Geometry check sheet. Reference: the model listing, model coordinates, mm. Face numbers are marked on the shaded views. A direction names the side the tool comes from. Give positions to 0.01 mm unless a question says otherwise; leave off trailing zeros. Order: outer loops, then holes, each group sorted by start corner. A loop starts at its lowest first (then second) coordinate and runs counter-clockwise, first axis right, second up. Notation, with made-up numbers: M -33.75,-29.75 L -19.75,-29.75 A12 ccw -19.75,-14.75 Z; hole C -25.75,-2.75 d2. An arc over 180 degrees is marked long. Answer as CSV lines item,"result".
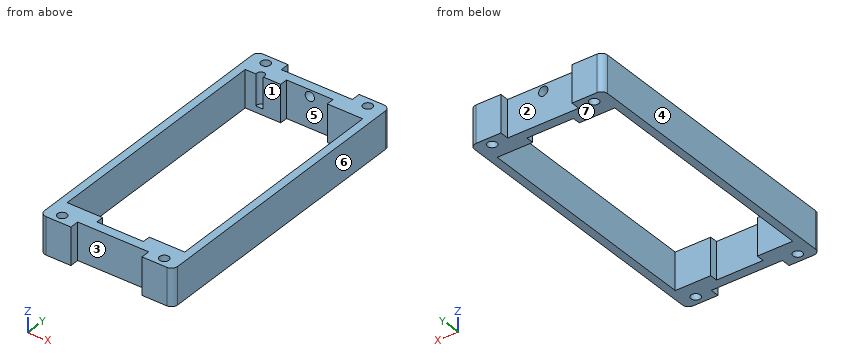
Autodesk Inventor part; units mm, degrees
ref_plane "YZ Plane" through (0, 0, 0) normal (1, 0, 0) x (0, 1, 0)
ref_plane "XZ Plane" through (0, 0, 0) normal (0, 1, 0) x (-1, 0, 0)
ref_plane "XY Plane" through (0, 0, 0) normal (0, 0, 1) x (1, 0, 0)
sketch "Эскиз1" plane through (0, 0, 0) normal (0, 0, 1) x (1, 0, 0)
  line L0 (-18.25, -37.6) -> (18.25, -37.6)
  line L1 (18.25, -37.6) -> (18.25, 37.6)
  line L2 (18.25, 37.6) -> (-18.25, 37.6)
  line L3 (-18.25, 37.6) -> (-18.25, -37.6)
  line L4 (-18.25, 0) -> (18.25, 0) construction
  line L5 (0, 37.6) -> (0, -37.6) construction
  line L6 (-18.45, -37.8) -> (18.45, -37.8)
  line L7 (18.45, -37.8) -> (18.45, 37.8)
  line L8 (18.45, 37.8) -> (-18.45, 37.8)
  line L9 (-18.45, 37.8) -> (-18.45, -37.8)
  line L10 (-7.5, -37.8) -> (7.5, -37.8)
  line L11 (7.5, -37.8) -> (7.5, -40.8)
  line L12 (7.5, -40.8) -> (-7.5, -40.8)
  line L13 (-7.5, -40.8) -> (-7.5, -37.8)
  line L14 (-18.45, -37.8) -> (-18.45, -43.8)
  line L15 (-18.45, -43.8) -> (18.45, -43.8)
  line L16 (18.45, -43.8) -> (18.45, -37.8)
  line L17 (-18.45, 43.8) -> (18.45, 43.8)
  line L18 (-18.45, 37.8) -> (-18.45, 43.8)
  line L19 (18.45, 43.8) -> (18.45, 37.8)
  line L20 (-18.45, -43.8) -> (-21.45, -43.8)
  line L21 (-21.45, -43.8) -> (-21.45, 43.8)
  line L22 (-21.45, 43.8) -> (-18.45, 43.8)
  line L23 (-18.45, 43.8) -> (-18.45, -43.8)
  line L24 (21.45, 43.8) -> (18.45, 43.8)
  line L25 (18.45, 37.8) -> (18.45, 43.8)
  line L26 (18.45, 43.8) -> (18.45, -43.8)
  line L27 (21.45, -43.8) -> (21.45, 43.8)
  line L28 (-7.5, 40.8) -> (-7.5, 37.8)
  line L29 (7.5, 40.8) -> (-7.5, 40.8)
  line L30 (7.5, 37.8) -> (7.5, 40.8)
  line L31 (-21.45, -43.8) -> (-11.45, -43.8)
  line L32 (18.45, -43.8) -> (21.45, -43.8)
  line L33 (21.45, -43.8) -> (11.45, -43.8)
  line L34 (16.45, 46.7) -> (21.45, 46.7)
  line L35 (16.45, 46.7) -> (11.45, 46.7)
  line L36 (11.45, 46.7) -> (11.45, 43.8)
  line L37 (21.45, 46.7) -> (21.45, 43.8)
  line L38 (11.45, 43.8) -> (16.45, 43.8)
  line L39 (-11.45, 46.7) -> (-11.45, 43.8)
  line L40 (-16.45, 46.7) -> (-11.45, 46.7)
  line L41 (-16.45, 46.7) -> (-21.45, 46.7)
  line L42 (-21.45, 46.7) -> (-21.45, 43.8)
  line L43 (-16.45, -46.7) -> (-21.45, -46.7)
  line L44 (-21.45, -46.7) -> (-21.45, -43.8)
  line L45 (-16.45, -46.7) -> (-11.45, -46.7)
  line L46 (-11.45, -46.7) -> (-11.45, -43.8)
  line L47 (11.45, -46.7) -> (11.45, -43.8)
  line L48 (16.45, -46.7) -> (11.45, -46.7)
  line L49 (16.45, -46.7) -> (21.45, -46.7)
  line L50 (21.45, -46.7) -> (21.45, -43.8)
  circle A0 centre (16.45, -43.8) radius 1.5
  circle A1 centre (-16.45, -43.8) radius 1.5
  circle A2 centre (16.45, 43.8) radius 1.5
  circle A3 centre (-16.45, 43.8) radius 1.5
  line L51 (0, 0) -> (-14.3, 0) construction
  line L52 (-14.3, 0) -> (-14.3, 38.8) construction
  line L53 (-14.3, 38.8) -> (0, 38.8) construction
  line L54 (0, 38.8) -> (0, 0) construction
  circle A4 centre (-14.3, 38.8) radius 1.25
  line L55 (18.45, -37.8) -> (18.95, -37.8)
  line L56 (18.95, -37.8) -> (18.95, -38.3)
  line L57 (18.95, -38.3) -> (18.45, -38.3)
  line L58 (18.45, -38.3) -> (18.45, -37.8)
  line L59 (18.95, -38.3) -> (-18.95, -38.3)
  line L60 (-18.95, -38.3) -> (-18.95, 38.3)
  line L61 (-18.95, 38.3) -> (18.95, 38.3)
  line L62 (18.95, 38.3) -> (18.95, -38.3)
  point P0 (-1.9914, -32.8601)
  point P1 (0, -37.8)
  point P2 (-15.05, 37.8)
  point P3 (-13.55, 37.8)
  point P4 (7.5, -38.3)
  point P5 (-7.5, -38.3)
  point P6 (-7.5, 38.3)
  point P7 (7.5, 38.3)
  dimension "d0" = 36.5
  dimension "d1" = 75.2
  dimension "d2" = 36.9
  dimension "d3" = 75.6
  dimension "d4" = 15
  dimension "d5" = 3
  dimension "d6" = 6
  dimension "d7" = 3
  dimension "d8" = 5
  dimension "d10" = 3
  dimension "d11" = 3
  dimension "d12" = 3
  dimension "d13" = 3
  dimension "d19" = 14.3
  dimension "d20" = 38.8
  dimension "d21" = 2.5
  dimension "d28" = 0.5
  dimension "d29" = 0.5
  dimension "d30" = 37.9
  dimension "d31" = 76.6
extrude "Выдавливание1" add sketch "Эскиз1" along normal blind 12 contours L61 L18 L17 A3 A2 L19 L30 L29 L28 A4 | A4 L61 | L61 L60 L59 L14 L20 L21 L22 L18 | L59 L13 L12 L11 L16 L15 A0 A1 L14 | L22 L42 L41 L40 L39 L17 A3 | L15 A1 L46 L45 L43 L44 L20 | L19 L24 L27 L32 L16 L57 L56 L62 L61 | L17 A2 L36 L35 L34 L37 L24 | L32 L50 L49 L48 L47 L15 A0
fillet "Сопряжение1" radius 2 4 edges at (-21.45, 46.7, 6) (21.45, 46.7, 6) (-21.45, -46.7, 6) (21.45, -46.7, 6)
extrude "Выдавливание3" cut sketch "Эскиз1" against normal blind 10 from surface at 12 contours A4 L61 L8 | A4 L61
sketch "Эскиз2" plane through (-11.45, 43.8, 0) normal (0, 1, 0) x (1, 0, 0)
  line L0 (32.9, 0) -> (32.9, -12) construction
  line L1 (32.9, -6) -> (-10, -6) construction
  line L2 (-10, -12) -> (-10, 0) construction
  line L3 (3.95, -12) -> (18.95, -12) construction
  line L4 (11.45, -12) -> (11.45, 0) construction
  line L5 (32.9, -12) -> (30.9, -12) construction
  line L6 (32.9, -12) -> (11.45, -12) construction
  line L7 (11.45, -12) -> (11.45, -9.9) construction
  line L8 (11.45, -9.9) -> (32.9, -9.9) construction
  line L9 (32.9, -9.9) -> (32.9, -12) construction
  circle A0 centre (11.45, -9.9) radius 1.5
  dimension "d24" = 2.1
  dimension "d25" = 3
extrude "Выдавливание4" cut sketch "Эскиз2" against normal blind 3
properties part number "fast_akkum2"
(1) Draft check along X on the marked faces 5, 6 and 7. Enter one of: +X half, -X half, draft (parallel to the pull), parting line (faces both ways), or undercut.
The answers:
face 5,"undercut"
face 6,"+X half"
face 7,"draft"
(2) Section check A-A on x = 10.5. Enter the section's corners in (y, z).
The answers:
outline,"M -43.8,0 L -38.3,0 L -38.3,12 L -43.8,12 Z; M 38.3,0 L 43.8,0 L 43.8,12 L 38.3,12 Z"
(3) Section check D-D on x = -16.45. Enter the section's corners in (y, z), then the cut area to 3 significant figures.
The answers:
outline,"M -46.7,0 L -45.3,0 L -45.3,12 L -46.7,12 Z; M -42.3,0 L -38.3,0 L -38.3,12 L -42.3,12 Z; M 38.3,0 L 42.3,0 L 42.3,12 L 38.3,12 Z; M 45.3,0 L 46.7,0 L 46.7,12 L 45.3,12 Z"
area,"130 mm2"
(4) Section check C-C on x = 0. Enter the section's corners in (y, z), then the cut area to 3 significant figures.
The answers:
outline,"M -43.8,0 L -40.8,0 L -40.8,12 L -43.8,12 Z; M 40.8,0 L 43.8,0 L 43.8,8.4 L 40.8,8.4 Z; M 40.8,11.4 L 43.8,11.4 L 43.8,12 L 40.8,12 Z"
area,"63.0 mm2"
(5) Section check B-B on y = -12.5. Enter the section's corners in (x, z), then the cut area to 3 significant figures.
The answers:
outline,"M -21.45,0 L -18.95,0 L -18.95,12 L -21.45,12 Z; M 18.95,0 L 21.45,0 L 21.45,12 L 18.95,12 Z"
area,"60.0 mm2"
(6) Material ranges on line 1 (Y direction, x = -16.45, z = 3); line 2 (X direction, y = -29, z = 3); line 3 (Y direction, x = -7, z = 8.75), recorded low to high.
The answers:
line 1,"y = -46.7 to -45.3, -42.3 to -38.3, 38.3 to 42.3, 45.3 to 46.7"
line 2,"x = -21.45 to -18.95, 18.95 to 21.45"
line 3,"y = -43.8 to -40.8, 40.8 to 43.8"
(7) Tool access check on the marked faces 1, 2, 3 and 4. Record the directions out of +Z, -Z, +X, -X, +Y, -Y that give a thin tool (end or side, any length) a straight path to the whole face; none if there is none.
The answers:
face 1,"+Z, -Z"
face 2,"+Z, -Z, +Y"
face 3,"+Z, -Z, -Y"
face 4,"+Z, -Z, -X, +Y, -Y"
(8) Gauge pin test, flat ends, axial feed: P1, Ø0.9, axis at y = -46, z = 4, coming from the +X side; P2, Ø5, axis at x = 0, z = 9.9, coming from the +Y side. Record the tip position at first contact, or that the pin passes through.
The answers:
P1,"stops at x = 21.26"
P2,"stops at y = 43.8"
